Geometry check sheet. Reference: the model listing, model coordinates, mm. Face numbers are marked on the shaded views. Round coordinates to 2 decimals unless told otherwise and drop trailing zeros. Loops run counter-clockwise (first coordinate to the right, second up) from the corner with the lowest first, then second, coordinate; pieces in that order, holes last. Notation, with made-up numbers: (74.5, 83.5) -> (106.5, 83.5) arc R15 ccw to (106.5, 90.5) -> close; hole circle Ø10 at (16, -32). An arc over 180 degrees is marked (long way). Use a Markdown table: item, result. Add a question column.
Q1. Release check for a two-part mould opening along Y. For the marked faces 1 and 2 record: released by +Y, released by -Y, zero draft, split by the parting line, or undercut.
Q2. Sectioned sample at B-B, the plane y = 2.45. Enter the section's corners in (x, z).
Q3. Sectioned sample at A-A, the plane z = 0. Enter the section's corners in (x, y).
Q4. Material ranges on L1, parallel to Y at x = 1.55, z = 0; L2, parallel to Z at x = 2.8, y = 1.55; L3, parallel to Y at x = 0.9, z = -0.75, recorded low to high.
Q5. Sectioned sample at C-C, the plane z = -2.1. Enter the section's corners in (x, y).
Q6. Gauge pin test, flat end, axial feed: P1, Ø1.2, axis at y = 0, z = 0, coming from the +X side. Record the tip position at first contact, or that the pin passes through.
Q7. Sectioned sample at D-D, the plane y = -1.45. Enter the section's corners in (x, z), then the cut area to 3 significant figures.
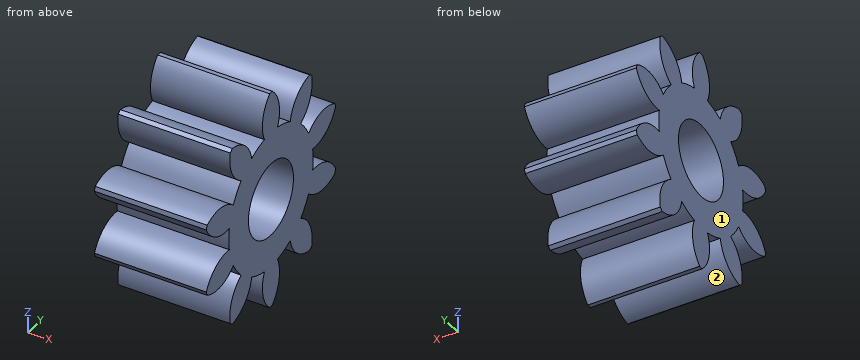
```python
from build123d import *

# Parameters (mm, degrees)
BASPROSKE_W           = 12
BASPROSKE_H           = 3
TOOTHCUT_DEPTH        = 13.727922061
TEETHCUTS_COUNT       = 10
TEETHCUTS_ANGLE       = 324
BORSKE_R              = 1
BORE_DEPTH            = 50.0000508
CROQUIS1_W            = 7.363545147
CROQUIS1_H            = 6.569840322
CORTAR_EXTRUIR1_DEPTH = 9


with BuildPart() as part:
    # BasProSke → Base-Revolve (revolve)
    with BuildSketch(Plane(origin=(0, 0, 0), x_dir=(1, 0, 0), z_dir=(0, 1, 0)), mode=Mode.PRIVATE) as base_revolve_sk:
        with Locations((6, 1.5)):
            Rectangle(BASPROSKE_W, BASPROSKE_H)
    revolve(base_revolve_sk.sketch.rotate(Axis((-10, 0, 0), (1, 0, 0)), 180), axis=Axis((-10, 0, 0), (1, 0, 0)))

    # TooCutSke → ToothCut (cut, through all)
    with BuildSketch(Plane(origin=(0, 0, 0), x_dir=(0, 0, -1), z_dir=(1, 0, 0))):
        with BuildLine():
            ThreePointArc((0.296449938, 1.850403587), (0, 1.874), (-0.296449938, 1.850403587))
            ThreePointArc((-0.296449938, 1.850403587), (-0.428089565, 2.470295585), (-0.905889751, 2.886591228))
            ThreePointArc((-0.905889751, 2.886591228), (0, 3.0254), (0.905889751, 2.886591228))
            ThreePointArc((0.905889751, 2.886591228), (0.428089565, 2.470295585), (0.296449938, 1.850403587))
        make_face()
    toothcut = extrude(amount=TOOTHCUT_DEPTH, mode=Mode.SUBTRACT)

    # TeethCuts: ToothCut ×10 about axis
    teethcuts_axis = Axis((-10, 0, 0), (1, 0, 0))
    for i in range(1, TEETHCUTS_COUNT):
        add(toothcut.rotate(teethcuts_axis, i * TEETHCUTS_ANGLE / (TEETHCUTS_COUNT - 1)), mode=Mode.SUBTRACT)

    # BorSke → Bore (cut, symmetric)
    with BuildSketch(Plane(origin=(0, 0, 0), x_dir=(0, 0, -1), z_dir=(1, 0, 0))):
        with Locations(Location((0, 0, 0), (0, 0, 180))):
            Circle(BORSKE_R)
    extrude(amount=BORE_DEPTH, both=True, mode=Mode.SUBTRACT)

    # Croquis1 → Cortar-Extruir1 (cut)
    with BuildSketch(Plane(origin=(12, 0, 0), x_dir=(0, 0, -1), z_dir=(1, 0, 0))):
        with Locations((0.087787386, 0.060578549)):
            Rectangle(CROQUIS1_W, CROQUIS1_H)
    extrude(amount=-CORTAR_EXTRUIR1_DEPTH, mode=Mode.SUBTRACT)


solid = part.part
```
Values:
| question | item | result |
|---|---|---|
| 1 | face 1 | zero draft |
| 1 | face 2 | undercut |
| 2 | outline | (0, -1.1) -> (3, -1.1) -> (3, -0.42) -> (0, -0.42) -> close; (0, 0.42) -> (3, 0.42) -> (3, 1.1) -> (0, 1.1) -> close |
| 3 | outline | (0, -1.87) -> (3, -1.87) -> (3, -1) -> (0, -1) -> close; (0, 1) -> (3, 1) -> (3, 1.87) -> (0, 1.87) -> close |
| 4 | L1 | -1.87 to -1, 1 to 1.87 |
| 4 | L2 | -2.43 to -1.5, -1.05 to 1.05, 1.5 to 2.43 |
| 4 | L3 | -2.8 to -0.66, 0.66 to 2.8 |
| 5 | outline | (0, -1.83) -> (3, -1.83) -> (3, -1.06) -> (0, -1.06) -> close; (0, -0.37) -> (3, -0.37) -> (3, 0.37) -> (0, 0.37) -> close; (0, 1.06) -> (3, 1.06) -> (3, 1.83) -> (0, 1.83) -> close |
| 6 | P1 | through |
| 7 | outline | (0, -2.39) -> (3, -2.39) -> (3, -1.41) -> (0, -1.41) -> close; (0, -1.19) -> (3, -1.19) -> (3, 1.19) -> (0, 1.19) -> close; (0, 1.41) -> (3, 1.41) -> (3, 2.39) -> (0, 2.39) -> close |
| 7 | area | 13.0 mm^2 |
